Geometry: final body of the model. Coordinates: model frame, mm. Face numbers are marked on the shaded views. A direction names the side the tool comes from. Give positions to 0.01 mm unless a question says otherwise; leave off trailing zeros. Order: outer loops, then holes, each group sorted by start corner. A loop starts at its lowest first (then second) coordinate and runs counter-clockwise, first axis right, second up. Notation, with made-up numbers: M 71.25,32.5 L 127.25,32.5 A25 cw 127.25,46.5 Z; hole C 78.25,-22 d1. An arc over 180 degrees is marked long. One line per item, written item: value. Start each with the question number.
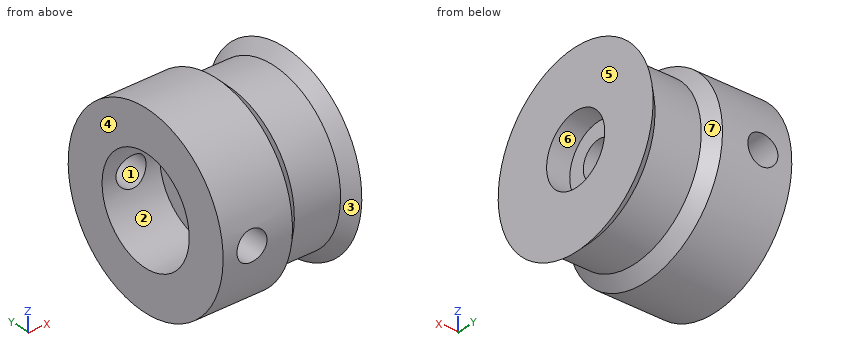
```python
from build123d import *

# Parameters (mm, degrees)
CUT_EXTRUDE1_DEPTH      = 17.492422502
CUT_EXTRUDE1_DEPTH_BACK = 17.492422502
SKETCH2_R               = 1.3
CHAMFER1_SIZE           = 1


with BuildPart() as part:
    # Sketch1 → Revolve1 (revolve)
    with BuildSketch(Plane.XY, mode=Mode.PRIVATE) as revolve1_sk:
        Polygon((0, 4.5), (0, 8), (7, 8), (7, 7), (11, 7), (11, 8), (12, 8), (12, 3), (10, 3), (10, 1.6), (5, 1.6), (5, 4.5), align=None)
    revolve(revolve1_sk.sketch.rotate(Axis((0, 0, 0), (1, 0, 0)), 90), axis=Axis((0, 0, 0), (1, 0, 0)))

    # Sketch2 → Cut-Extrude1 (cut, two sides: drawn at the far end of the back side and taken through both)
    with BuildSketch(Plane(origin=(0, 0, 0), x_dir=(1, 0, 0), z_dir=(0, 1, 0)).offset(-CUT_EXTRUDE1_DEPTH_BACK)):
        with Locations(Location((2.5, 0, 0), (0, 0, 270))):
            Circle(SKETCH2_R)
    extrude(amount=CUT_EXTRUDE1_DEPTH + CUT_EXTRUDE1_DEPTH_BACK, mode=Mode.SUBTRACT)

    # Chamfer1
    chamfer1_edges = [part.edges().sort_by_distance(p)[0] for p in [
        (11, 0, -8),
        (7, 0, -8),
    ]]
    chamfer(chamfer1_edges, length=CHAMFER1_SIZE - 0.0001)  # a hair under: the kernel refuses the full size


solid = part.part
```
Q1. Section query B-B on x = 3.25. Return loops of the section in (y, z), and give its area (4 significant figures).
Q2. Ray query, line 1 along Y through (x, z) = (8.6, 0); line 2 along X through (y, z) = (7.1, 0); line 3 along Z through (x, y) = (2.5, 6.7). Return the intervals inside material, ascending. Write a range as [from, to].
Q3. Mould query, pull axis X, two halves, no side actions, for the marked faces 4, 5, 6 and 7. Classes: +X half, -X half, draft (parallel to the pull), parting line (faces both ways), or undercut.
Q4. Section query D-D on x = 8.25. Return loops of the section in (y, z).
Q5. Section query C-C on z = 0. Give the number of separate pieces and of enclosed holes in the cut face, and give its area (3 significant figures).
Q6. Set-up query: the marked faces 1, 2 and 3. Return all of +Z, -Z, +X, -X, +Y, -Y with unobstructed straight access to the full face (end or side cutting, diameter ignored); none if empty.
Q7. Contact query for flat-ended pins moving along their axis: pin 1 (1 mm diameter, centred on x = 7, y = 3, fed in from +Z); pin 2 (1 mm diameter, centred on x = 8.5, z = 5.5, fed in from -Y); pin 3 (1.5 mm diameter, centred on x = 9.5, z = -3, fed in from -Y). Output: stop coordinate, or through.
Results below:
1. outline: M -7.93,-1.06 A8 ccw 7.93,-1.06 L 4.37,-1.06 A4.5 cw -4.37,-1.06 Z; M -7.93,1.06 L -4.37,1.06 A4.5 cw 4.37,1.06 L 7.93,1.06 A8 ccw Z
1. area: 122.5 mm2
2. line 1: [-7, -1.6], [1.6, 7]
2. line 2: [0, 1.2], [3.8, 6.9], [11.1, 12]
2. line 3: [-4.37, -1.3], [1.3, 4.37]
3. face 4: -X half
3. face 5: +X half
3. face 6: draft
3. face 7: undercut
4. outline: C 0,0 d14; hole C 0,0 d3.2
5. separate pieces: 4
5. enclosed holes: 0
5. area: 90.8 mm2
6. face 1: +Y, -Y
6. face 2: -X
6. face 3: none
7. pin 1: z = 6.91
7. pin 2: y = -4.9
7. pin 3: y = -6.63
